The listing builds one solid part. Answer for the finished solid, in the listing's coordinates (mm). A direction names the side the tool comes from. Coordinates: 2 decimals unless noted, no trailing zeros. Loops run counter-clockwise (first coordinate to the right, second up) from the corner with the lowest first, then second, coordinate; pieces in that order, holes last. Notation, with made-up numbers: M -33.5,38 L -6.5,38 A19 ccw -6.5,68 Z; hole C 15.25,30.5 d11. An arc over 180 degrees is marked long. Answer as a JSON object with one key per item and string values. Group by question number.
1. A cutting plane is placed at B-B on x = 3. Give the vertices of the cut face in (y, z).
2. A cutting plane is placed at C-C on y = 0. State how many separate pieces and enclosed holes the cut face has, and give its area (3 significant figures).
3. Determine the mould class of faces 5 (the face through (39.04, 5.862, 2.969)), 6 (the face through (0, 9, 6)), 7 (the face through (40.821, 13.662, 2.969)) for opening direction X: released by +X, released by -X, zero draft, split by the parting line, or undercut.
4. For faces 1 (the face through (44.39, 3.77, 0.41)), 2 (the face through (62, -2, 2)), 3 (the face through (-39.01, 5.87, 2.97)), 4 (the face through (-44.29, 3.84, 5.61)), determine the directions among +Z, -Z, +X, -X, +Y, -Y from which every point of the face is accessible in a straight line to the end or side of a thin tool.
5. Straight lines are drawn through the part: L1, parallel to Y at x = -60, z = 4.7; L2, parallel to Y at x = -60, z = 0.8; L3, parallel to X at y = -1.5, z = 2.5. For each, find the intervals that lie inside material, in ascending order.
6. A cutting plane is placed at A-A on x = -60. Give the vertices of the cut face in (y, z).
7. Given pin 1 (2 mm diameter, centred on x = 15.5, z = 4.5, fed in from -Y); pin 2 (3.5 mm diameter, centred on x = 60, y = 0, fed in from +Z); pin 3 (3.5 mm diameter, centred on x = -59, y = 0, fed in from +Z); pin 4 (2 mm diameter, centred on y = 5.5, z = 4, fed in from +X), each flat-ended and moving along its own axis, determine where each tip first touches the part or whether it passes through.
from build123d import *

# Parameters (mm, degrees)
SKETCH1_R           = 2.05
BOSS_EXTRUDE1_DEPTH = 6
SKETCH3_R           = 3.6
CUT_EXTRUDE1_DEPTH  = 4
CHAMFER3_SIZE       = 0.8


with BuildPart() as part:
    # Sketch1 → Boss-Extrude1 (new body)
    with BuildSketch(Plane.XY):
        with BuildLine():
            Line((-51.788854382, 8.577708764), (-43.689164944, 12.627553483))
            ThreePointArc((-43.689164944, 12.627553483), (-40.86217617, 13.652236863), (-37.875388203, 14))
            Line((-37.875388203, 14), (37.875388203, 14))
            ThreePointArc((37.875388203, 14), (40.86217617, 13.652236863), (43.689164944, 12.627553483))
            Line((43.689164944, 12.627553483), (51.788854382, 8.577708764))
            ThreePointArc((51.788854382, 8.577708764), (54.213536442, 7.949847309), (56.683281573, 8.366563146))
            ThreePointArc((56.683281573, 8.366563146), (68.049844719, -4.024922359), (51.316718427, -2.366563146))
            ThreePointArc((51.316718427, -2.366563146), (50.168244018, -0.140737539), (48.211145618, 1.422291236))
            Line((48.211145618, 1.422291236), (40.11145618, 5.472135955))
            ThreePointArc((40.11145618, 5.472135955), (39.024152805, 5.866244947), (37.875388203, 6))
            Line((37.875388203, 6), (-37.875388203, 6))
            ThreePointArc((-37.875388203, 6), (-39.024152805, 5.866244947), (-40.11145618, 5.472135955))
            Line((-40.11145618, 5.472135955), (-48.211145618, 1.422291236))
            ThreePointArc((-48.211145618, 1.422291236), (-50.168244018, -0.140737539), (-51.316718427, -2.366563146))
            ThreePointArc((-51.316718427, -2.366563146), (-68.049844719, -4.024922359), (-56.683281573, 8.366563146))
            ThreePointArc((-56.683281573, 8.366563146), (-54.213536442, 7.949847309), (-51.788854382, 8.577708764))
        make_face()
        with Locations((-60, 0)):
            Circle(SKETCH1_R, mode=Mode.SUBTRACT)
        with Locations((60, 0)):
            Circle(SKETCH1_R, mode=Mode.SUBTRACT)
    extrude(amount=BOSS_EXTRUDE1_DEPTH)

    # Sketch3 → Cut-Extrude1 (cut)
    with BuildSketch(Plane.XY.offset(6)):
        with Locations((-60, 0)):
            Circle(SKETCH3_R)
        with Locations((60, 0)):
            Circle(SKETCH3_R)
    extrude(amount=-CUT_EXTRUDE1_DEPTH, mode=Mode.SUBTRACT)

    # Chamfer3
    chamfer3_edges = [part.edges().sort_by_distance(p)[0] for p in [
        (-40.86217617, 13.652236863, 6),
        (47.739009663, 10.602631123, 0),
        (54.213536442, 7.949847309, 0),
        (68.049844719, -4.024922359, 0),
        (-47.739009663, 10.602631123, 6),
        (50.168244018, -0.140737539, 0),
        (44.161300899, 3.447213595, 0),
        (39.024152805, 5.866244947, 0),
        (0, 6, 0),
        (-39.024152805, 5.866244947, 0),
        (-44.161300899, 3.447213595, 0),
        (-50.168244018, -0.140737539, 0),
        (-68.049844719, -4.024922359, 0),
        (-54.213536442, 7.949847309, 0),
        (-47.739009663, 10.602631123, 0),
        (-54.213536442, 7.949847309, 6),
        (-40.86217617, 13.652236863, 0),
        (0, 14, 0),
        (40.86217617, 13.652236863, 0),
        (-68.049844719, -4.024922359, 6),
        (-50.168244018, -0.140737539, 6),
        (-44.161300899, 3.447213595, 6),
        (-39.024152805, 5.866244947, 6),
        (0, 6, 6),
        (39.024152805, 5.866244947, 6),
        (44.161300899, 3.447213595, 6),
        (40.86217617, 13.652236863, 6),
        (50.168244018, -0.140737539, 6),
        (68.049844719, -4.024922359, 6),
        (54.213536442, 7.949847309, 6),
        (47.739009663, 10.602631123, 6),
        (0, 14, 6),
    ]]
    chamfer(chamfer3_edges, length=CHAMFER3_SIZE)


solid = part.part
From the geometry:
{
 "1": {"outline": "M 6,0.8 L 6.8,0 L 13.2,0 L 14,0.8 L 14,5.2 L 13.2,6 L 6.8,6 L 6,5.2 Z"},
 "2": {"separate pieces": "4", "enclosed holes": "0", "area": "150 mm²"},
 "3": {"face 5": "undercut", "face 6": "zero draft", "face 7": "released by +X"},
 "4": {"face 1": "-Z, -Y", "face 2": "+Z", "face 3": "+Z, -Z, -Y", "face 4": "+Z, -Y"},
 "5": {"L1": "y = -9 to -3.6, 3.6 to 9", "L2": "y = -9 to -2.05, 2.05 to 9", "L3": "x = -68.87 to -63.27, -56.73 to -51.01, 51.01 to 56.73, 63.27 to 68.87"},
 "6": {"outline": "M -9,0.8 L -8.2,0 L -2.05,0 L -2.05,2 L -3.6,2 L -3.6,6 L -8.2,6 L -9,5.2 Z; M 2.05,0 L 8.2,0 L 9,0.8 L 9,5.2 L 8.2,6 L 3.6,6 L 3.6,2 L 2.05,2 Z"},
 "7": {"pin 1": "stops at y = 6", "pin 2": "passes through", "pin 3": "stops at z = 2", "pin 4": "stops at x = 67.79"}
}
